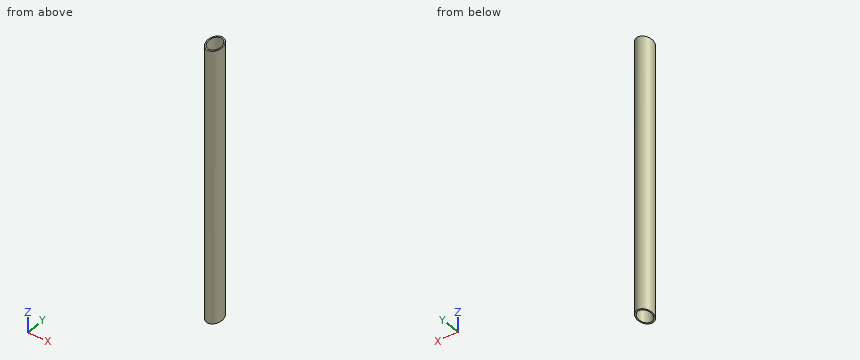
Autodesk Inventor part; units mm, degrees
ref_plane "Start Plane" through (0, 0, -33.777) normal (0, 0, 1) x (1, 0, 0)
ref_plane "End Plane" through (0, 0, 787.5852) normal (0, 0, 1) x (1, 0, 0)
ref_plane "Work Plane4" through (3.0414, 5.4547, -23.3078) normal (0.126, 0.2261, -0.9659) x (0.5338, -0.8362, -0.126)
ref_plane "Start Plane" through (0, 0, -33.777) normal (0, 0, 1) x (1, 0, 0)
ref_plane "End Plane" through (0, 0, 787.5852) normal (0, 0, 1) x (1, 0, 0)
sketch "Sketch" plane through (0, 0, 0) normal (0, 0, 1) x (1, 0, 0)
  circle A0 centre (0, 0) radius 20.447
  circle A1 centre (0, 0) radius 24.13
  dimension "d0" = 48.26
  dimension "d1" = 3.683
extrude "Body" add sketch "Sketch" along normal up to surface (821.3622 mm away) from surface at -33.777
sketch "Sketch3" plane through (0, 0, 0) normal (0, 0, 1) x (1, 0, 0)
  line L0 (0, 0) -> (10, 0)
ref_plane "Work Plane3" through (0, 0, 0) normal (0, -1, 0) x (1, 0, 0)
ref_plane "Work Plane4" through (3.0414, 5.4547, -23.3078) normal (0.126, 0.2261, -0.9659) x (0.5338, -0.8362, -0.126)
split "Split1" plane through (3.0414, 5.4547, -23.3078) removes the side toward (0.126, 0.2261, -0.9659)
ref_plane "Work Plane5" through (3.1674, 5.6807, 780.5322) normal (-0.126, -0.2261, 0.9659) x (0.9919, -0.0145, 0.126)
split "Split2" plane through (3.1674, 5.6807, 780.5322) removes the side toward (-0.126, -0.2261, 0.9659)
sketch "Sketch4" plane through (0, 0, 0) normal (0, -1, 0) x (1, 0, 0)
  line L0 (-2, -33.777) -> (12, -33.777)
  line L1 (-2, 787.5852) -> (12, 787.5852)
  dimension "d7" = 821.3622
equation "\"d0\" = G_H"
equation "\"d1\" = G_T"
equation "\"d2\" = G_L"
equation "\"G_H\" = 48.26"
equation "\"G_T\" = 3.683"
equation "\"G_L\" = d7"
equation "\"G_OFFSET_START\" = 33.77702"
equation "\"G_OFFSET_END\" = -17.22068"
equation "\"d4\" = -G_OFFSET_START"
equation "\"d5\" = G_OFFSET_END + B_L"
equation "\"B_L\" = 804.8059"
properties part number "ANSI - 1 1/2 x 0.145 - 32.337" material "Steel, Mild"
Build history of the part. All positions in model axes, mm. Give positions to 0.01 mm unless a question says otherwise; leave off trailing zeros. Write each loop counter-clockwise with the first axis right and the second up, starting at its lowest first coordinate (ties: lowest second). Pieces come first, ordered by that corner, then holes. Notation, with made-up numbers: (-29.75, 6.5) - (-0.75, 6.5) arc R18 ccw to (-0.75, 13.5) - close; hole circle Ø2 at (61, 11). An arc over 180 degrees is marked (long way). Use one line per item in the form item = value. Start each with the question number.
1. Band-saw the part on B-B on y = 13. Write the cut outline in (x, z).
2. Probe line 1 (X direction, y = 0, z = 139); line 2 (X direction, y = 2, z = 457.5). List the from-to ranges inside material, lowest first. Write a range as [from, to].
3. Drop flat-ended pins along their axis: pin 1 Ø12 at (y, z) = (10.5, 468.5) entering from +X; pin 2 Ø8 at (x, z) = (19, 654.5) entering from +Y; pin 3 Ø8 at (x, z) = (5.5, 560) entering from -Y; pin 4 Ø24.5 at (x, y) = (0, 0) entering from -Z. Give the stop position or say it passes through.
4. Band-saw the part on A-A on x = -11. Write the cut outline in (y, z).
5. Band-saw the part on C-C on z = 391.5. Write the cut outline in (x, y).
Conclusion:
q1.outline = (-20.33, -24.59) - (-15.78, -24) - (-15.78, 779.77) - (-20.33, 779.18) - close; (15.78, -19.88) - (20.33, -19.29) - (20.33, 784.48) - (15.78, 783.89) - close
q2.line_1 = [-24.13, -20.45], [20.45, 24.13]
q2.line_2 = [-24.05, -20.35], [20.35, 24.05]
q3.pin_1 = 23.71
q3.pin_2 = 18.9
q3.pin_3 = -24.08
q3.pin_4 = through
q4.outline = (-21.48, -31.44) - (-17.24, -30.45) - (-17.24, 773.32) - (-21.48, 772.33) - close; (17.24, -22.38) - (21.48, -21.39) - (21.48, 782.38) - (17.24, 781.39) - close
q5.outline = circle Ø48.26 at (0, 0); hole circle Ø40.89 at (0, 0)
